```python
from build123d import *

# Parameters (mm, degrees)
F0_W     = 10
F0_H     = 10
F0_W_2   = 11
F1_DEPTH = 20
F2_W     = 10.5
F2_H     = 10
F3_DEPTH = 10
F4_DEPTH = 20


with BuildPart() as f1:
    # F0 (on Front) → F1 (new body)
    with BuildSketch(Plane.XZ):
        with Locations((-24.396219, 5.872731)):
            Rectangle(F0_W, F0_H)
        with Locations((-13.896219, 5.872731)):
            Rectangle(F0_W_2, F0_H)
    extrude(amount=F1_DEPTH)

    # F2 (on face) → F3 (cut)
    with BuildSketch(Plane.XZ.offset(20)):
        with Locations((-13.646219, 5.872731)):
            Rectangle(F2_W, F2_H)
    extrude(amount=-F3_DEPTH, mode=Mode.SUBTRACT)

    # F0 (on Front) → F4 (join)
    with BuildSketch(Plane.XZ):
        with Locations((-3.396219, 5.872731)):
            Rectangle(F0_W, F0_H)
    extrude(amount=F4_DEPTH)


solid = f1.part
```
Geometry check sheet. Reference: the model listing, model coordinates, mm. A direction names the side the tool comes from. Round coordinates to 2 decimals unless told otherwise and drop trailing zeros. Loops run counter-clockwise (first coordinate to the right, second up) from the corner with the lowest first, then second, coordinate; pieces in that order, holes last. Notation, with made-up numbers: M -26.75,47.25 L -5.75,47.25 A33 cw -5.75,82.25 Z; hole C 46,40 d7. An arc over 180 degrees is marked long. Return JSON: item names as keys, results as strings. Group by question number.
(1) Section check C-C, the plane x = -15. Enter the section's corners in (y, z).
(2) Section check B-B, the plane z = 6. Enter the section's corners in (x, y).
(3) Scan lines: line 1 along X through (y, z) = (-10.5, 6.25); line 2 along Y through (x, z) = (-18, 1.5). Record each from-to range of solid material in increasing order. Write a range as [from, to].
(4) Go/stop test with a flat-tipped pin: pin 1 (5 mm diameter, centred on x = -14.5, z = 6.5, fed in from -Y). Record where the tip stops, or that it passes through.
(5) Section check A-A, the plane y = -16.75. Enter the section's corners in (x, z), and give its area (3 significant figures).
(6) Set-up check for faces 1 (the face through (-18.896, -15, 6)), 2 (the face through (-29.396, -10, 6)): record each of +Z, -Z, +X, -X, +Y, -Y from which the full face is reachable in a straight line by a thin tool's end or side.
Data:
{
 "1": {"outline": "M -10,0.87 L 0,0.87 L 0,10.87 L -10,10.87 Z"},
 "2": {"outline": "M -29.4,-20 L -18.9,-20 L -18.9,-10 L -8.4,-10 L -8.4,-20 L 1.6,-20 L 1.6,0 L -29.4,0 Z"},
 "3": {"line 1": "[-29.4, -18.9], [-8.4, 1.6]", "line 2": "[-10, 0]"},
 "4": {"pin 1": "y = -10"},
 "5": {"outline": "M -29.4,0.87 L -18.9,0.87 L -18.9,10.87 L -29.4,10.87 Z; M -8.4,0.87 L 1.6,0.87 L 1.6,10.87 L -8.4,10.87 Z", "area": "205 mm²"},
 "6": {"face 1": "+Z, -Z, -Y", "face 2": "+Z, -Z, -X, +Y, -Y"}
}
